from build123d import *

# Parameters (mm, degrees)
RESSALTO_EXTRUS_O1_DEPTH = 20
CASCA1_T                 = -3
ESBO_O2_W                = 2
ESBO_O2_H                = 89
RESSALTO_EXTRUS_O2_DEPTH = 17
ESBO_O3_R                = 4
CORTE_EXTRUS_O1_DEPTH    = 111.440028975
ESBO_O4_R                = 4
CORTE_EXTRUS_O2_DEPTH    = 44
CORTE_EXTRUS_O3_DEPTH    = 2


with BuildPart() as part:
    # Esboço1 → Ressalto-extrusão1 (new body)
    with BuildSketch(Plane.XY):
        with BuildLine():
            Line((-58, 23), (-58, 68))
            Line((-58, 68), (-82, 68))
            Line((-82, 68), (-82, -52))
            ThreePointArc((-82, -52), (-76.142135624, -66.142135624), (-62, -72))
            Line((-62, -72), (62, -72))
            ThreePointArc((62, -72), (76.142135624, -66.142135624), (82, -52))
            Line((82, -52), (82, 68))
            Line((82, 68), (58, 68))
            Line((58, 68), (58, 23))
            Line((58, 23), (9.5, 23))
            Line((9.5, 23), (9.5, 30))
            Line((9.5, 30), (-9.5, 30))
            Line((-9.5, 30), (-9.5, 23))
            Line((-9.5, 23), (-58, 23))
        make_face()
    extrude(amount=RESSALTO_EXTRUS_O1_DEPTH)

    # Casca1
    casca1_openings = [part.faces().sort_by_distance(p)[0] for p in [
        (0, -15.157706838, 20),
    ]]
    offset(amount=CASCA1_T, openings=casca1_openings, kind=Kind.INTERSECTION)

    # Esboço2 → Ressalto-extrusão2 (add)
    with BuildSketch(Plane.XY.offset(3)):
        with Locations((-23, -24.5)):
            Rectangle(ESBO_O2_W, ESBO_O2_H)
        with Locations((23, -24.5)):
            Rectangle(ESBO_O2_W, ESBO_O2_H)
    extrude(amount=RESSALTO_EXTRUS_O2_DEPTH)

    # Esboço3 → Corte-extrusão1 (cut, through all)
    with BuildSketch(Plane.XY.offset(3)):
        with Locations((70, 55)):
            Circle(ESBO_O3_R)
    extrude(amount=-CORTE_EXTRUS_O1_DEPTH, mode=Mode.SUBTRACT)

    # Esboço4 → Corte-extrusão2 (cut)
    with BuildSketch(Plane.XY.offset(3)):
        with Locations((-70, 55)):
            Circle(ESBO_O4_R)
    extrude(amount=-CORTE_EXTRUS_O2_DEPTH, mode=Mode.SUBTRACT)

    # Esboço5 → Corte-extrusão3 (cut)
    with BuildSketch(Plane.XY.offset(20)):
        with BuildLine():
            Line((-8.5, 22), (-59, 22))
            Line((-59, 22), (-59, 67))
            Line((-59, 67), (-81, 67))
            Line((-81, 67), (-81, -52))
            ThreePointArc((-81, -52), (-75.435028843, -65.435028843), (-62, -71))
            Line((-62, -71), (62, -71))
            ThreePointArc((62, -71), (75.435028843, -65.435028843), (81, -52))
            Line((81, -52), (81, 67))
            Line((81, 67), (59, 67))
            Line((59, 67), (59, 22))
            Line((59, 22), (8.5, 22))
            Line((8.5, 22), (8.5, 29))
            Line((8.5, 29), (-8.5, 29))
            Line((-8.5, 29), (-8.5, 22))
        make_face()
        with BuildLine():
            Line((-62, -70), (62, -70))
            ThreePointArc((62, -70), (74.727922061, -64.727922061), (80, -52))
            Line((80, -52), (80, 66))
            Line((80, 66), (60, 66))
            Line((60, 66), (60, 21))
            Line((60, 21), (7.5, 21))
            Line((7.5, 21), (7.5, 28))
            Line((7.5, 28), (-7.5, 28))
            Line((-7.5, 28), (-7.5, 21))
            Line((-7.5, 21), (-60, 21))
            Line((-60, 21), (-60, 66))
            Line((-60, 66), (-80, 66))
            Line((-80, 66), (-80, -52))
            ThreePointArc((-80, -52), (-74.727922061, -64.727922061), (-62, -70))
        make_face(mode=Mode.SUBTRACT)
    extrude(amount=-CORTE_EXTRUS_O3_DEPTH, mode=Mode.SUBTRACT)


solid = part.part
Geometry check sheet. Reference: the model listing, model coordinates, mm. A direction names the side the tool comes from. Give positions to 0.01 mm unless a question says otherwise; leave off trailing zeros. Loops run counter-clockwise (first coordinate to the right, second up) from the corner with the lowest first, then second, coordinate; pieces in that order, holes last. Notation, with made-up numbers: M 12.5,62.5 L 60.5,62.5 A32 cw 60.5,89.5 Z; hole C -32,0 d11. An arc over 180 degrees is marked long. Answer as a JSON object with one key per item and string values. Group by question number.
Item 1: Sectioned sample at B-B on x = -56. Record the boundary of the cut face in (y, z), plus the area to 3 significant figures.
Item 2: Sectioned sample at D-D on z = 8. Give the number of separate pieces and of enclosed holes in the cut face, plus the area to 3 significant figures.
Item 3: Access from +Z, -Z, +X, -X, +Y, -Y to the whole of each face (thin tool, end or side, straight path). Record for faces 4 (the flat face through (-70, 68, 10)), 5 (the flat face through (58, 46, 10)), 6 (the flat face through (0, 27, 11)).
Item 4: Mould release check, pull along Y, two halves, no side actions. Record for faces 1 (the cylindrical face through (75.986, -66.297, 9.86)), 2 (the flat face through (70, 68, 10)), 3 (the cylindrical face through (74.587, -64.867, 19.014)): pulls with the +Y half, pulls with the -Y half, needs draft (parallel to the pull), parting line crosses it, or undercut.
Item 5: Material ranges on L1, parallel to X at y = -25.5, z = 5.75; L2, parallel to X at y = 48.5, z = 11; L3, parallel to Y at x = 32, z = 11, recorded low to high.
Item 6: Sectioned sample at C-C on y = -9.5. Record the boundary of the cut face in (x, z).
Item 7: Gauge pin test, flat ends, axial feed: pin 1 (2 mm diameter, centred on x = 3.5, z = 18.5, fed in from +Y); pin 2 (6 mm diameter, centred on x = 34, z = 17, fed in from +Y). Record the tip position at first contact, or that the pin passes through.
Findings below:
{
 "1": {"outline": "M -72,0 L 23,0 L 23,20 L 22,20 L 22,18 L 21,18 L 21,20 L 20,20 L 20,3 L -69,3 L -69,20 L -70,20 L -70,18 L -71,18 L -71,20 L -72,20 Z", "area": "383 mm2"},
 "2": {"separate pieces": "1", "enclosed holes": "3", "area": "2,410 mm2"},
 "3": {"face 4": "+Z, -Z, +X, -X, +Y", "face 5": "+Z, -Z, +Y", "face 6": "+Z"},
 "4": {"face 1": "pulls with the -Y half", "face 2": "pulls with the +Y half", "face 3": "undercut"},
 "5": {"L1": "-82 to -79, -24 to -22, 22 to 24, 79 to 82", "L2": "-82 to -79, -61 to -58, 58 to 61, 79 to 82", "L3": "-72 to -69, 20 to 23"},
 "6": {"outline": "M -82,0 L 82,0 L 82,20 L 81,20 L 81,18 L 80,18 L 80,20 L 79,20 L 79,3 L 24,3 L 24,20 L 22,20 L 22,3 L -22,3 L -22,20 L -24,20 L -24,3 L -79,3 L -79,20 L -80,20 L -80,18 L -81,18 L -81,20 L -82,20 Z"},
 "7": {"pin 1": "y = 30", "pin 2": "y = 23"}
}
